Read the model definition and answer for the solid it produces. Units are mm, in the model's axes. A direction names the side the tool comes from. Coordinates: 2 decimals unless noted, no trailing zeros. Write each loop counter-clockwise with the first axis right and the second up, starting at its lowest first coordinate (ties: lowest second). Pieces come first, ordered by that corner, then holes. Notation, with made-up numbers: (23.25, -19) -> (37.25, -19) arc R27 ccw to (37.25, 7) -> close; hole circle Ø8 at (77, -30.75). An arc over 180 degrees is marked (long way). Answer as a JSON object with one key per item and string values. Group by question number.
(1) Straight lines are drawn through the part: L1, parallel to Y at x = 0.5, z = 1.45; L2, parallel to Z at x = 4.25, y = 2.25; L3, parallel to Y at x = 3.25, z = 1.2. For each, find the intervals that lie inside material, in ascending order.
(2) For a pull along Y with two mould halves and no side action, classify faces 4 (the face through (3, 12.5, 1.2)), 5 (the face through (3, 7.5, 1.2)), 6 (the face through (3, 17.5, 1.2)), 7 (the face through (3, 11, 1.5)) as +Y half, -Y half, draft (parallel to the pull), parting line (faces both ways), or undercut.
(3) Find section D-D (x = 2.25). Give the vertices of the cut face in (y, z) (3 decimals).
(4) Find section C-C (y = 10.25). Give the vertices of the cut face in (x, z).
(5) Find section B-B (x = 5). Give the vertices of the cut face in (y, z).
(6) Which of the six approach directions +Z, -Z, +X, -X, +Y, -Y give full straight-line access (tool end or side, diameter ignored) to faces 1 (the face through (3, 20, 0.5)), 2 (the face through (4, 19, 1)), 3 (the face through (3, 15, 1.2))?
(7) Find section A-A (y = 18.25). Give the vertices of the cut face in (x, z), then the cut area to 3 significant figures.
Autodesk Fusion 360 part; units mm, degrees
sketch "Sketch1" plane through (0, 0, 0) normal (0, 0, 1) x (1, 0, 0)
  line L0 (0, 0) -> (6, 0)
  line L1 (6, 0) -> (6, 20)
  line L2 (6, 20) -> (0, 20)
  line L3 (0, 20) -> (0, 0)
  dimension "d1" = 6
  dimension "d2" = 20
extrude "Extrude1" add sketch "Sketch1" along normal blind 1 makes body 1
sketch "Sketch2" plane through (0, 0, 1) normal (0, 0, 1) x (-1, 0, 0)
  line L0 (0, -20) -> (0, 0)
  line L1 (0, 0) -> (-6, 0)
  line L2 (-6, 0) -> (-6, -20)
  line L3 (-6, -20) -> (0, -20)
  line L4 (0, -20) -> (-6, -15)
  line L5 (0, -15) -> (-6, -10)
  line L6 (0, -10) -> (-6, -5)
  line L7 (0, -5) -> (-6, 0)
  line L8 (0, -7.5) -> (-6, -2.4178)
  line L9 (0, -12.5) -> (-6, -7.5)
  line L10 (0, -17.5) -> (-6, -12.5)
extrude "Extrude2" add sketch "Sketch2" along normal blind 0.5 contours L0 L2 L4 L10 | L0 L2 L5 L9 | L0 L2 L6 L8 | L0 L1 L7 bodies 1
copy_body "Body->Comp1" bodies 1 removing the originals makes body 2 in component "Component"
component "Component" placed x (1, 0, 0) y (0, 1, 0) z (0, 0, 1) at (0, 0, 0)
Results below:
{
 "1": {"L1": "y = 0 to 4.58, 7.08 to 9.58, 12.08 to 14.58, 17.08 to 19.58", "L2": "z = 0 to 1", "L3": "y = 0 to 2.29, 4.75 to 7.29, 9.79 to 12.29, 14.79 to 17.29"},
 "2": {"face 4": "undercut", "face 5": "undercut", "face 6": "+Y half", "face 7": "draft"},
 "3": {"outline": "(0, 0) -> (20, 0) -> (20, 1) -> (18.125, 1) -> (18.125, 1.5) -> (15.625, 1.5) -> (15.625, 1) -> (13.125, 1) -> (13.125, 1.5) -> (10.625, 1.5) -> (10.625, 1) -> (8.125, 1) -> (8.125, 1.5) -> (5.594, 1.5) -> (5.594, 1) -> (3.125, 1) -> (3.125, 1.5) -> (0, 1.5) -> close"},
 "4": {"outline": "(0, 0) -> (6, 0) -> (6, 1) -> (5.7, 1) -> (5.7, 1.5) -> (2.7, 1.5) -> (2.7, 1) -> (0, 1) -> close"},
 "5": {"outline": "(0, 0) -> (20, 0) -> (20, 1) -> (15.83, 1) -> (15.83, 1.5) -> (13.33, 1.5) -> (13.33, 1) -> (10.83, 1) -> (10.83, 1.5) -> (8.33, 1.5) -> (8.33, 1) -> (5.83, 1) -> (5.83, 1.5) -> (3.26, 1.5) -> (3.26, 1) -> (0.83, 1) -> (0.83, 1.5) -> (0, 1.5) -> close"},
 "6": {"face 1": "+Z, -Z, +X, -X, +Y", "face 2": "+Z, +X, +Y", "face 3": "+Z"},
 "7": {"outline": "(0, 0) -> (6, 0) -> (6, 1) -> (2.1, 1) -> (2.1, 1.5) -> (0, 1.5) -> close", "area": "7.05 mm2"}
}
